Autodesk Inventor part; units mm, degrees
ref_plane "YZ Plane" through (0, 0, 0) normal (1, 0, 0) x (0, 1, 0)
ref_plane "XZ Plane" through (0, 0, 0) normal (0, 1, 0) x (-1, 0, 0)
ref_plane "XY Plane" through (0, 0, 0) normal (0, 0, 1) x (1, 0, 0)
sketch "Sketch1" plane through (0, 0, 0) normal (0, 0, 1) x (1, 0, 0)
  line L0 (0, 0) -> (15, 0)
  line L1 (15, 0) -> (15, 70)
  line L2 (15, 70) -> (0, 70)
  line L3 (0, 70) -> (0, 0)
  line L4 (15, 35) -> (0, 35)
  line L5 (0, 60) -> (15, 60)
  line L6 (15, 60) -> (15, 10)
  line L7 (15, 10) -> (0, 10)
  line L8 (0, 10) -> (0, 60)
  line L9 (0, 60) -> (15, 10) construction
  line L10 (15, 60) -> (0, 10) construction
  line L11 (7.5, 35) -> (8, 35)
  circle A0 centre (8, 35) radius 5.15
  line L12 (0, 0) -> (15, 0)
  line L13 (15, 0) -> (15, 15)
  line L14 (15, 15) -> (0, 15) construction
  line L15 (0, 15) -> (0, 0)
  line L16 (0, 70) -> (15, 70)
  line L17 (15, 70) -> (15, 55)
  line L18 (15, 55) -> (0, 55) construction
  line L19 (0, 55) -> (0, 70)
  line L20 (15, 15) -> (0, 0) construction
  line L21 (0, 70) -> (15, 55) construction
  circle A1 centre (7.5, 7.5) radius 7.5
  circle A2 centre (7.5, 62.5) radius 7.5
  line L22 (0, 10) -> (15, 10)
  line L23 (15, 10) -> (15, 25)
  line L24 (15, 25) -> (0, 25)
  line L25 (0, 25) -> (0, 10)
  line L26 (15, 60) -> (0, 60)
  line L27 (0, 60) -> (0, 45)
  line L28 (0, 45) -> (15, 45)
  line L29 (15, 45) -> (15, 60)
  line L30 (0, 45) -> (15, 60) construction
  line L31 (0, 10) -> (15, 25) construction
  circle A3 centre (7.5, 17.5) radius 4
  circle A4 centre (7.5, 52.5) radius 4
  circle A5 centre (7.5, 7.5) radius 4.05
  circle A6 centre (7.5, 62.5) radius 4.05
  point P0 (15, 7.5)
  point P1 (15, 62.5)
  point P2 (0, 62.5)
  point P3 (0, 7.5)
  point P4 (7.5, 70)
  point P5 (7.5, 0)
  dimension "d0" = 15
  dimension "d1" = 70
  dimension "d2" = 15
  dimension "d3" = 50
  dimension "d5" = 0.5
  dimension "d6" = 10.3
  dimension "d7" = 15
  dimension "d8" = 15
  dimension "d9" = 15
  dimension "d10" = 15
  dimension "d11" = 15
  dimension "d12" = 15
  dimension "d13" = 15
  dimension "d14" = 15
  dimension "d15" = 8
  dimension "d16" = 8
  dimension "d26" = 8.1
  dimension "d27" = 8.1
extrude "Extrusion1" add sketch "Sketch1" against normal blind 15 contours A3 A1 | A1 A3 | A4 A2 | A2 A4
extrude "Extrusion2" add sketch "Sketch1" along normal blind 15 contours L3 A1 L0 | A1 L1 L0 | A1 L7 A5 | L3 L7 A1 | A1 L7 L1 | L3 L24 L1 L7 A1 A3 | A1 A3 L7 A5 | A3 A1 | A1 A3 | L3 L4 A0 L1 L24 | L3 L28 L1 L4 A0 | L3 L5 A2 A4 L1 L28 | L3 A2 L5 | L5 A2 L1 | L3 L2 A2 | A2 L5 A6 | L5 A6 A2 A4 | A2 L2 L1 | A4 A2 | A2 A4
fillet "Fillet2" radius 7.5 4 edges at (15, 0, 7.5) (0, 0, 7.5) (15, 70, 7.5) (0, 70, 7.5)
chamfer "Chamfer2" distance 2 angle 45 12 edges at (12.8033, 67.8033, 15) (12.8033, 2.1967, 15) (2.1967, 67.8033, 15) (2.1967, 2.1967, 15) (0, 35, 15) (15, 35, 15) (15, 35, 0) (12.8033, 67.8033, 0) (12.8033, 2.1967, 0) (2.1967, 67.8033, 0) (2.1967, 2.1967, 0) (0, 35, 0)
properties part number "Gear_Holder_1"
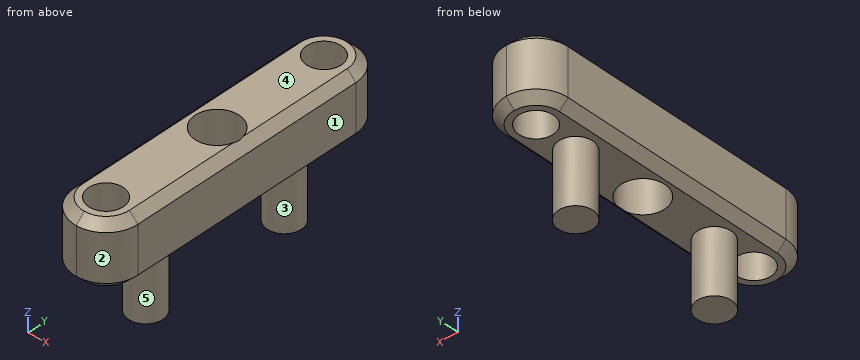
Geometry: final body of the model. Coordinates: model frame, mm. Face numbers are marked on the shaded views. A direction names the side the tool comes from. Give positions to 0.01 mm unless a question says otherwise; leave off trailing zeros. Write each loop counter-clockwise with the first axis right and the second up, starting at its lowest first coordinate (ties: lowest second). Pieces come first, ordered by that corner, then holes. Notation, with made-up numbers: (3, -20) -> (16, -20) arc R15 ccw to (16, -3) -> close; hole circle Ø5 at (61.25, -13). An arc over 180 degrees is marked (long way). Answer in a Markdown table with one row per item.
(1) Pin query (flat end, axial travel): pin 1 (10 mm diameter, centred on y = 60, z = -6, fed in from +X); pin 2 (12 mm diameter, centred on y = 8, z = 6, fed in from -X); pin 3 (6.5 mm diameter, centred on x = 7.5, y = 62.5, fed in from -Z); pin 4 (1 mm diameter, centred on x = 2.5, z = 7.5, fed in from -Y). Return the tip coordinate at first contact, or that it passes through.
Answers below:
| item | result |
|---|---|
| pin 1 | x = 10.62 |
| pin 2 | x = 0 |
| pin 3 | through |
| pin 4 | y = 1.5 |
(2) Ray query, line 1 along Y through (x, z) = (8, 3); line 2 along Y through (x, z) = (6.25, 5.5); line 3 along Y through (x, z) = (7.75, -9.75). Return the intervals inside material, ascending. Write a range as [from, to].
Answers below:
| item | result |
|---|---|
| line 1 | [0.02, 3.48], [11.52, 29.85], [40.15, 58.48], [66.52, 69.98] |
| line 2 | [0.1, 3.65], [11.35, 30.16], [39.84, 58.65], [66.35, 69.9] |
| line 3 | [13.51, 21.49], [48.51, 56.49] |
(3) Section query A-A on y = 35. Return loops of the section in (x, z), then the cut area to 3 significant figures.
Answers below:
| item | result |
|---|---|
| outline | (0, 2) -> (2, 0) -> (2.85, 0) -> (2.85, 15) -> (2, 15) -> (0, 13) -> close; (13.15, 0.15) -> (15, 2) -> (15, 13) -> (13.15, 14.85) -> close |
| area | 62.5 mm^2 |
(4) Set-up query: the marked faces 4 and 5. Return all of +Z, -Z, +X, -X, +Y, -Y with unobstructed straight access to the full face (end or side cutting, diameter ignored); none if empty.
Answers below:
| item | result |
|---|---|
| face 4 | +Z, +X, -X, +Y, -Y |
| face 5 | -Z |
(5) Section query D-D on y = 17.5. Return loops of the section in (x, z).
Answers below:
| item | result |
|---|---|
| outline | (0, 2) -> (2, 0) -> (3.5, 0) -> (3.5, -15) -> (11.5, -15) -> (11.5, 0) -> (13, 0) -> (15, 2) -> (15, 13) -> (13, 15) -> (2, 15) -> (0, 13) -> close |
(6) Section query B-B on z = 8.25. State how many separate pieces and enclosed holes the cut face has, then the cut area to 3 significant figures.
Answers below:
| item | result |
|---|---|
| separate pieces | 1 |
| enclosed holes | 3 |
| area | 815 mm^2 |
(7) Draft query along Y for the marked faces 1, 2 and 3. Return one class per face: +Y half, -Y half, draft (parallel to the pull), parting line (faces both ways), or undercut.
Answers below:
| item | result |
|---|---|
| face 1 | draft |
| face 2 | -Y half |
| face 3 | undercut |
(8) Section query C-C on z = -8. Return loops of the section in (x, y), then the cut area to 3 significant figures.
Answers below:
| item | result |
|---|---|
| outline | circle Ø8 at (7.5, 17.5); circle Ø8 at (7.5, 52.5) |
| area | 101 mm^2 |
